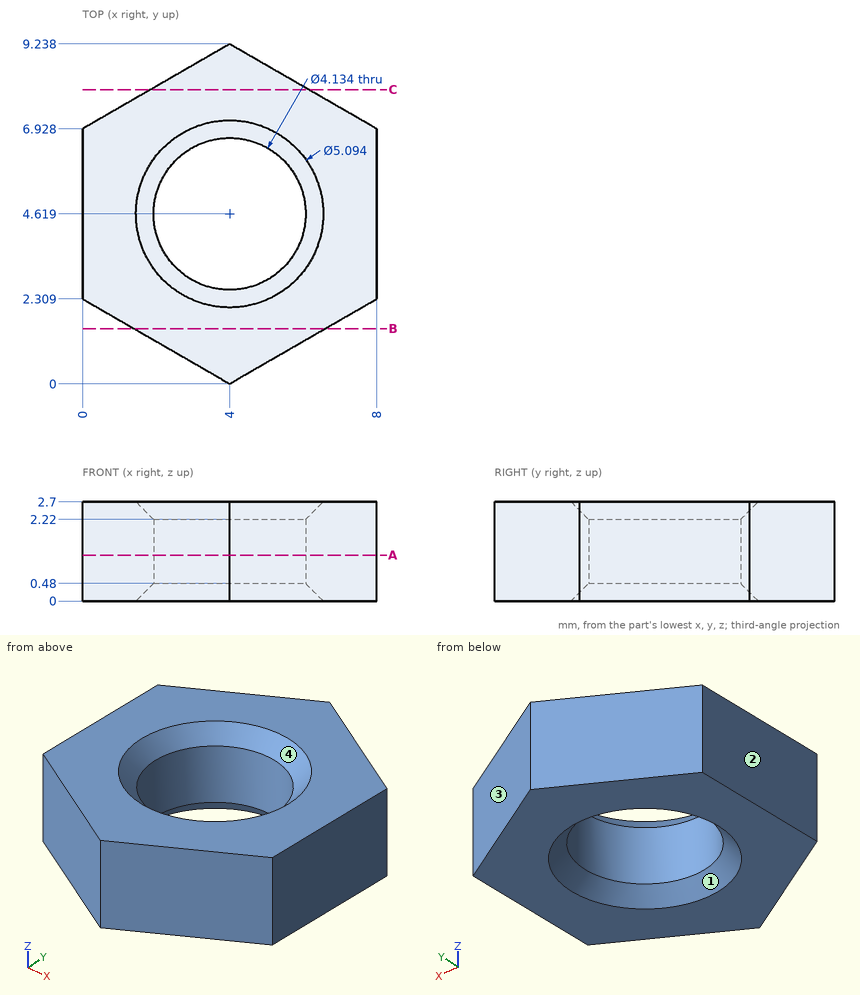
Input: dimensioned drawing with shaded views. Units: mm. Origin: part minimum x, y, z. Round coordinates to 2 decimals unless told otherwise and drop trailing zeros. Loops run counter-clockwise (first coordinate to the right, second up) from the corner with the lowest first, then second, coordinate; pieces in that order, holes last. Notation, with made-up numbers: (54, 24.25) -> (103, 24.25) arc R17 ccw to (103, 33.25) -> close; hole circle Ø6 at (-38.75, -21.75). An arc over 180 degrees is marked (long way). Answer as a JSON object with one key per item and string values. Group by question number.
Q1. Contact query for flat-ended pins moving along their axis: P1, Ø1.5, axis at x = 3, z = 2, coming from the -Y side (1 decimal); P2, Ø1, axis at x = 5, z = 1.5, coming from the -Y side; P3, Ø4, axis at x = 3.5, y = 6.5, coming from the +Z side. Output: stop coordinate, or through.
Q2. Ray query, line 1 (Y direction, x = 4.25, z = 0.7) (1 decimal); line 2 (X direction, y = 5.5, z = 1.7); line 3 (X direction, y = 4.75, z = 1.1). Return the intervals inside material, ascending. Write a range as from..to.
Q3. Mould query, pull axis Y, two halves, no side actions, for the marked faces 1, 2, 3 and 4. Classes: pulls with the +Y half, pulls with the -Y half, needs draft (parallel to the pull), parting line crosses it, or undercut.
Q4. Section query C-C (y = 8). Output: boundary loops of the cut face in (x, z).
Q5. Section query B-B (y = 1.5). Output: boundary loops of the cut face in (x, z).
Q6. Section query A-A (z = 1.25). Output: boundary loops of the cut face in (x, y).
Completed:
{
 "1": {"P1": "y = 0.1", "P2": "y = 0.29", "P3": "z = 2.7"},
 "2": {"line 1": "0.1..2.6, 6.7..9.1", "line 2": "0..2.13, 5.87..8", "line 3": "0..1.94, 6.06..8"},
 "3": {"face 1": "undercut", "face 2": "needs draft", "face 3": "pulls with the +Y half", "face 4": "undercut"},
 "4": {"outline": "(1.86, 0) -> (6.14, 0) -> (6.14, 2.7) -> (1.86, 2.7) -> close"},
 "5": {"outline": "(1.4, 0) -> (6.6, 0) -> (6.6, 2.7) -> (1.4, 2.7) -> close"},
 "6": {"outline": "(0, 2.31) -> (4, 0) -> (8, 2.31) -> (8, 6.93) -> (4, 9.24) -> (0, 6.93) -> close; hole circle Ø4.13 at (4, 4.62)"}
}
